```python
from build123d import *

# Parameters (mm, degrees)
SKETCH1_W           = 130
SKETCH1_H           = 80
SKETCH1_W_2         = 110
SKETCH1_H_2         = 60
BOSS_EXTRUDE2_DEPTH = 200
SKETCH4_W           = 130
SKETCH4_H           = 80
BOSS_EXTRUDE3_DEPTH = 10
SKETCH6_R           = 28.535717896
SKETCH6_R_2         = 19.989594855
BOSS_EXTRUDE5_DEPTH = 75
CUT_EXTRUDE1_START  = -75
SKETCH6_3_R         = 19.989594855
CUT_EXTRUDE1_DEPTH  = 75


with BuildPart() as part:
    # Sketch1 → Boss-Extrude2 (new body)
    with BuildSketch(Plane.XY):
        with Locations((65, -40)):
            Rectangle(SKETCH1_W, SKETCH1_H)
        with Locations((65, -40)):
            Rectangle(SKETCH1_W_2, SKETCH1_H_2, mode=Mode.SUBTRACT)
    extrude(amount=BOSS_EXTRUDE2_DEPTH)

    # Sketch4 → Boss-Extrude3 (add)
    with BuildSketch(Plane.XY.offset(200)):
        with Locations((65, -40)):
            Rectangle(SKETCH4_W, SKETCH4_H)
    extrude(amount=BOSS_EXTRUDE3_DEPTH)

    # Sketch6 → Boss-Extrude5 (add)
    with BuildSketch(Plane(origin=(130, 0, 0), x_dir=(0, 0, -1), z_dir=(1, 0, 0))):
        with Locations(Location((-35.002467087, -39.78091539, 0), (0, 0, 180))):
            Circle(SKETCH6_R)
        with Locations((-35.002467087, -39.78091539)):
            Circle(SKETCH6_R_2, mode=Mode.SUBTRACT)
    extrude(amount=BOSS_EXTRUDE5_DEPTH)

    # Sketch6_3 → Cut-Extrude1 (cut)
    with BuildSketch(Plane(origin=(130, 0, 0), x_dir=(0, 0, -1), z_dir=(1, 0, 0)).offset(CUT_EXTRUDE1_START)):
        with Locations(Location((-35.002467087, -39.78091539, 0), (0, 0, 270))):
            Circle(SKETCH6_3_R)
    extrude(amount=CUT_EXTRUDE1_DEPTH, mode=Mode.SUBTRACT)


solid = part.part
```
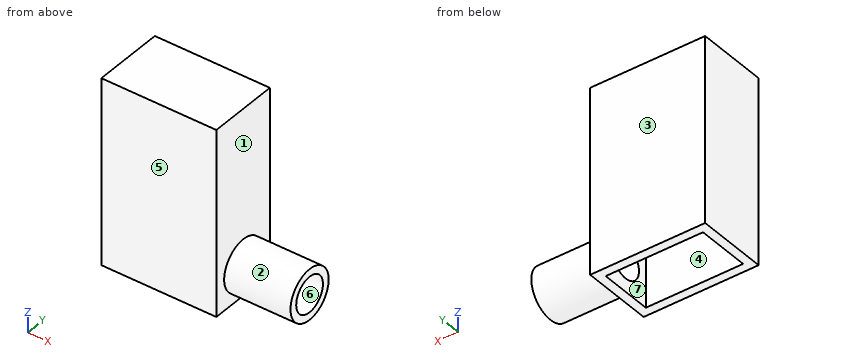
Source: CAD feature listing. Evaluate the final solid. Frame: model axes, mm. Face numbers are marked on the shaded views. A direction names the side the tool comes from. Coordinates: 2 decimals unless noted, no trailing zeros. Write each loop counter-clockwise with the first axis right and the second up, starting at its lowest first coordinate (ties: lowest second). Pieces come first, ordered by that corner, then holes. Notation, with made-up numbers: (35.5, -33.5) -> (65.5, -33.5) arc R18 cw to (65.5, -26.5) -> close; hole circle Ø8 at (80.25, 69.5). An arc over 180 degrees is marked (long way). Return JSON: item names as keys, results as strings. Group by question number.
1) Section query A-A, the plane z = 101. Return loops of the section in (x, y), plus the area to 3 significant figures.
2) Ray query, line 1 along Y through (x, z) = (104, 194); line 2 along X through (y, z) = (-56, 140); line 3 along Z through (x, y) = (114.5, -20). Return the intervals inside material, ascending.
3) Section query B-B, the plane y = -26.5. Return loops of the section in (x, z), plus the area to 3 significant figures.
4) Section query C-C, the plane x = 77. Return loops of the section in (y, z).
5) Section query D-D, the plane y = -56. Return loops of the section in (x, z).
6) Set-up query: the marked faces 5, 6 and 7. Return all of +Z, -Z, +X, -X, +Y, -Y with unobstructed straight access to the full face (end or side cutting, diameter ignored); none if empty.
7) Mould query, pull axis Y, two halves, no side actions, for the marked faces 1, 2, 3 and 4. Classes: +Y half, -Y half, draft (parallel to the pull), parting line (faces both ways), or undercut.
8) Contact query for flat-ended pins moving along their axis: P1, Ø8, axis at y = -22.5, z = 110, coming from the +X side; P2, Ø1, axis at x = 59, y = -61, coming from the -Z side. Output: stop coordinate, or through.
From the geometry:
{
 "1": {"outline": "(0, -80) -> (130, -80) -> (130, 0) -> (0, 0) -> close; hole (10, -70) -> (120, -70) -> (120, -10) -> (10, -10) -> close", "area": "3,800 mm²"},
 "2": {"line 1": "-80 to -70, -10 to 0", "line 2": "0 to 10, 120 to 130", "line 3": "200 to 210"},
 "3": {"outline": "(0, 0) -> (10, 0) -> (10, 200) -> (120, 200) -> (120, 49.94) -> (205, 49.94) -> (205, 60.26) -> (130, 60.26) -> (130, 210) -> (0, 210) -> close; (120, 0) -> (130, 0) -> (130, 9.75) -> (205, 9.75) -> (205, 20.06) -> (120, 20.06) -> close", "area": "6,550 mm²"},
 "4": {"outline": "(-80, 0) -> (-70, 0) -> (-70, 200) -> (-10, 200) -> (-10, 0) -> (0, 0) -> (0, 210) -> (-80, 210) -> close"},
 "5": {"outline": "(0, 0) -> (10, 0) -> (10, 200) -> (120, 200) -> (120, 46.69) -> (205, 46.69) -> (205, 58.48) -> (130, 58.48) -> (130, 210) -> (0, 210) -> close; (120, 0) -> (130, 0) -> (130, 11.52) -> (205, 11.52) -> (205, 23.32) -> (120, 23.32) -> close"},
 "6": {"face 5": "+Z, -Z, +X, -X, -Y", "face 6": "+X", "face 7": "-Z"},
 "7": {"face 1": "draft", "face 2": "parting line", "face 3": "+Y half", "face 4": "undercut"},
 "8": {"P1": "x = 130", "P2": "z = 200"}
}
